Work out the finished part from the listing and answer in its coordinate system (mm). A direction names the side the tool comes from. Round coordinates to 2 decimals unless told otherwise and drop trailing zeros. Order: outer loops, then holes, each group sorted by start corner. A loop starts at its lowest first (then second) coordinate and runs counter-clockwise, first axis right, second up. Notation, with made-up numbers: M -5.75,19 L 46.25,19 A28 ccw 46.25,47 Z; hole C 1.5,31.25 d1. An arc over 180 degrees is marked long. Return JSON: item names as keys, results as strings.
from build123d import *

# Parameters (mm, degrees)
F0_W     = 34
F0_H     = 21
F1_DEPTH = 5
F0_W_2   = 24
F0_H_2   = 8.5
F0_H_3   = 2.5
F2_DEPTH = 3
F3_DEPTH = 2.5
F4_R     = 1.1
F5_DEPTH = 3
F6_R     = 1.25
F7_DEPTH = 8


with BuildPart() as f1:
    # F0 (on Top) → F1 (new body)
    with BuildSketch(Plane.XY):
        with Locations((-17, 10.5)):
            Rectangle(F0_W, F0_H)
        Polygon((-29, 13.5), (-29, 16), (-5, 16), (-5, 13.5), (-5, 5), (-29, 5), align=None, mode=Mode.SUBTRACT)
    extrude(amount=F1_DEPTH)

    # F0 (on Top) → F2 (join)
    with BuildSketch(Plane.XY):
        with Locations((-17, 10.5)):
            Rectangle(F0_W, F0_H)
        Polygon((-29, 13.5), (-29, 16), (-5, 16), (-5, 13.5), (-5, 5), (-29, 5), align=None, mode=Mode.SUBTRACT)
        with Locations((-17, 9.25)):
            Rectangle(F0_W_2, F0_H_2)
        with Locations((-17, 14.75)):
            Rectangle(F0_W_2, F0_H_3)
    extrude(amount=-F2_DEPTH)

    # F0 (on Top) → F3 (cut)
    with BuildSketch(Plane.XY):
        with Locations((-17, 14.75)):
            Rectangle(F0_W_2, F0_H_3)
    extrude(amount=-F3_DEPTH, mode=Mode.SUBTRACT)

    # F4 (on face) → F5 (cut, through all)
    with BuildSketch(Plane.XY):
        with Locations((-26.2, 7.8)):
            Circle(F4_R)
    extrude(amount=-F5_DEPTH, mode=Mode.SUBTRACT)

    # F6 (on face) → F7 (cut, through all)
    with BuildSketch(Plane.XY.offset(5)):
        with Locations((-31.5, 18.5)):
            Circle(F6_R)
        with Locations((-2.5, 18.5)):
            Circle(F6_R)
        with Locations((-2.5, 2.5)):
            Circle(F6_R)
        with Locations((-31.5, 2.5)):
            Circle(F6_R)
    extrude(amount=-F7_DEPTH, mode=Mode.SUBTRACT)


solid = f1.part
Item 1: Which of the six approach directions +Z, -Z, +X, -X, +Y, -Y give full straight-line access (tool end or side, diameter ignored) to faces 1 (the flat face through (-17, 0, 1)), 2 (the flat face through (-17, 15, -2.5))?
Output:
{"face 1": "+Z, -Z, +X, -X, -Y", "face 2": "+Z"}
Item 2: Find section B-B (x = -2.5). Determine the outline of the cut face in (y, z).
Output:
{"outline": "M 0,-3 L 1.25,-3 L 1.25,5 L 0,5 Z; M 3.75,-3 L 17.25,-3 L 17.25,5 L 3.75,5 Z; M 19.75,-3 L 21,-3 L 21,5 L 19.75,5 Z"}
Item 3: Find section C-C (z = 2). Determine the outline of the cut face in (x, y), plus the area to 3 significant figures.
Output:
{"outline": "M -34,0 L 0,0 L 0,21 L -34,21 Z; hole C -31.5,2.5 d2.5; hole C -31.5,18.5 d2.5; hole M -29,5 L -5,5 L -5,16 L -29,16 Z; hole C -2.5,2.5 d2.5; hole C -2.5,18.5 d2.5", "area": "430 mm^2"}
Item 4: Consider line 1 along Y through (x, z) = (-31.5, 0.5); line 2 along Y through (x, z) = (-8.5, 1.75); line 3 along Y through (x, z) = (-26.2, -0.6). Determine where each line is inside the solid, lowest interval first. Write a range as [from, to].
Output:
{"line 1": "y = [0, 1.25], [3.75, 17.25], [19.75, 21]", "line 2": "y = [0, 5], [16, 21]", "line 3": "y = [0, 6.7], [8.9, 13.5], [16, 21]"}
Item 5: The mould has two halves that part along X. Classify faces 3 (the flat face through (-34, 10, 1)), 4 (the flat face through (0, 10, 1)), 5 (the flat face through (-5, 11, 2)): pulls with the +X half, pulls with the -X half, needs draft (parallel to the pull), parting line crosses it, or undercut.
Output:
{"face 3": "pulls with the -X half", "face 4": "pulls with the +X half", "face 5": "undercut"}
Item 6: Each of these flat-tipped pins is pushed along its axis until it touches: pin 1 (7 mm diameter, centred on x = -15, y = 11.5, fed in from +Z); pin 2 (1.2 mm diameter, centred on x = -16, y = 15, fed in from +Z); pin 3 (2 mm diameter, centred on x = -26.2, y = 7.8, fed in from -Z) (3 decimals). Where does it stop, or does it pass through?
Output:
{"pin 1": "stops at z = 0", "pin 2": "stops at z = -2.5", "pin 3": "passes through"}
Item 7: Find section D-D (x = -26.2). Determine the outline of the cut face in (y, z), plus the area to 3 significant figures.
Output:
{"outline": "M 0,-3 L 6.7,-3 L 6.7,0 L 5,0 L 5,5 L 0,5 Z; M 8.9,-3 L 21,-3 L 21,5 L 16,5 L 16,-2.5 L 13.5,-2.5 L 13.5,0 L 8.9,0 Z", "area": "100 mm^2"}
Item 8: Find section A-A (y = 7.8). Determine the outline of the cut face in (x, z), plus the area to 3 significant figures.
Output:
{"outline": "M -34,-3 L -27.3,-3 L -27.3,0 L -29,0 L -29,5 L -34,5 Z; M -25.1,-3 L 0,-3 L 0,5 L -5,5 L -5,0 L -25.1,0 Z", "area": "145 mm^2"}
